Autodesk Inventor part; units mm, degrees
ref_plane "NUT_XY" through (0, 0, 0) normal (0, 0, 1) x (1, 0, 0)
ref_plane "NUT_YZ" through (0, 0, 0) normal (1, 0, 0) x (0, 1, 0)
ref_plane "NUT_ZX" through (0, 0, 0) normal (0, 1, 0) x (0, 0, 1)
sketch "Sketch_8" plane through (0, 0, 0) normal (1, 0, 0) x (0, 1, 0)
  line L0 (0, -3.048) -> (0, 0)
  line L1 (0, 0) -> (4.7625, 0)
  line L2 (4.7625, 0) -> (5.715, -0.2552)
  line L3 (5.715, -0.2552) -> (5.715, -2.7928)
  line L4 (5.715, -2.7928) -> (4.7625, -3.048)
  line L5 (4.7625, -3.048) -> (0, -3.048)
  line L6 (0, -3.048) -> (0, 0)
sketch "Sketch_10" plane through (0, 0, 0) normal (0, 0, 1) x (1, 0, 0)
  line L0 (-9.525, -9.525) -> (9.525, -9.525)
  line L1 (9.525, -9.525) -> (9.525, 9.525)
  line L2 (9.525, 9.525) -> (-9.525, 9.525)
  line L3 (-9.525, 9.525) -> (-9.525, -9.525)
  line L4 (-4.7625, -2.7496) -> (0, -5.4993)
  line L5 (0, -5.4993) -> (4.7625, -2.7496)
  line L6 (4.7625, -2.7496) -> (4.7625, 2.7496)
  line L7 (4.7625, 2.7496) -> (0, 5.4993)
  line L8 (0, 5.4993) -> (-4.7625, 2.7496)
  line L9 (-4.7625, 2.7496) -> (-4.7625, -2.7496)
revolve "Revolution1" add sketch "Sketch_8" angle 360 about axis through (0, 0, -3.048) along (0, 0, -1)
extrude "Extrusion1" cut sketch "Sketch_10" against normal blind 3.048
sketch "Sketch_11" plane through (0, 0, 0) normal (1, 0, 0) x (0, 1, 0)
  line L0 (0, -3.048) -> (0, 0)
  line L1 (0, 0) -> (2.413, 0)
  line L2 (2.413, 0) -> (1.9837, -0.4293)
  line L3 (1.9837, -0.4293) -> (1.9837, -2.6187)
  line L4 (1.9837, -2.6187) -> (2.413, -3.048)
  line L5 (2.413, -3.048) -> (0, -3.048)
  line L6 (0, -3.048) -> (0, 0)
revolve "Revolution2" cut sketch "Sketch_11" angle 360 about axis through (0, 0, -3.048) along (0, 0, -1)
thread "Thread1"
ref_plane "NUT_XY" through (0, 0, 0) normal (0, 0, 1) x (1, 0, 0)
ref_plane "NUT_YZ" through (0, 0, 0) normal (1, 0, 0) x (0, 1, 0)
ref_plane "NUT_ZX" through (0, 0, 0) normal (0, 1, 0) x (0, 0, 1)
ref_plane "a1_XY" through (-4.7625, 4.7625, 0) normal (0, 0, 1) x (1, 0, 0)
ref_plane "a1_YZ" through (-4.7625, 4.7625, 0) normal (1, 0, 0) x (0, 1, 0)
ref_plane "a1_ZX" through (-4.7625, 4.7625, 0) normal (0, 1, 0) x (0, 0, 1)
ref_plane "a2_XY" through (4.7625, 4.7625, 0) normal (0, 0, 1) x (1, 0, 0)
ref_plane "a2_YZ" through (4.7625, 4.7625, 0) normal (1, 0, 0) x (0, 1, 0)
ref_plane "a2_ZX" through (4.7625, 4.7625, 0) normal (0, 1, 0) x (0, 0, 1)
ref_plane "b1_XY" through (0, 4.7625, 0) normal (1, 0, 0) x (0, 0, -1)
ref_plane "b1_YZ" through (0, 4.7625, 0) normal (0, 0, -1) x (0, 1, 0)
ref_plane "b1_ZX" through (0, 4.7625, 0) normal (0, 1, 0) x (1, 0, 0)
ref_plane "b2_XY" through (0, 4.7625, -3.048) normal (1, 0, 0) x (0, 0, -1)
ref_plane "b2_YZ" through (0, 4.7625, -3.048) normal (0, 0, -1) x (0, 1, 0)
ref_plane "b2_ZX" through (0, 4.7625, -3.048) normal (0, 1, 0) x (1, 0, 0)
ref_plane "e_XY" through (0, 0, -3.048) normal (1, 0, 0) x (0, 0, -1)
ref_plane "e_YZ" through (0, 0, -3.048) normal (0, 0, -1) x (0, 1, 0)
ref_plane "e_ZX" through (0, 0, -3.048) normal (0, 1, 0) x (1, 0, 0)
ref_plane "ol1_XY" through (0, 0, -4.7625) normal (0, 1, 0) x (1, 0, 0)
ref_plane "ol1_YZ" through (0, 0, -4.7625) normal (1, 0, 0) x (0, 0, -1)
ref_plane "ol1_ZX" through (0, 0, -4.7625) normal (0, 0, -1) x (0, 1, 0)
ref_plane "ol2_XY" through (3.048, 0, -4.7625) normal (0, 1, 0) x (1, 0, 0)
ref_plane "ol2_YZ" through (3.048, 0, -4.7625) normal (1, 0, 0) x (0, 0, -1)
ref_plane "ol2_ZX" through (3.048, 0, -4.7625) normal (0, 0, -1) x (0, 1, 0)
ref_plane "th1_XY" through (0, 2.413, -3.048) normal (1, 0, 0) x (0, 0, -1)
ref_plane "th1_YZ" through (0, 2.413, -3.048) normal (0, 0, -1) x (0, 1, 0)
ref_plane "th1_ZX" through (0, 2.413, -3.048) normal (0, 1, 0) x (1, 0, 0)
ref_plane "th2_XY" through (0, -2.413, -3.048) normal (1, 0, 0) x (0, 0, -1)
ref_plane "th2_YZ" through (0, -2.413, -3.048) normal (0, 0, -1) x (0, 1, 0)
ref_plane "th2_ZX" through (0, -2.413, -3.048) normal (0, 1, 0) x (1, 0, 0)
properties part number "D-5288"
CAD build for the part. Positions are in the model's coordinates, mm. Coordinates: 2 decimals unless noted, no trailing zeros. Order: outer loops, then holes, each group sorted by start corner. A loop starts at its lowest first (then second) coordinate and runs counter-clockwise, first axis right, second up. Notation, with made-up numbers: M -31,44 L 7,44 A15 ccw 7,73 Z; hole C -4,-33.5 d3. An arc over 180 degrees is marked long. Answer as CSV lines item,"result".
1) Cut at A-A (z = -1.35). List the corners of the cut face in (x, y), then the cut area to 3 significant figures.
Verdict:
outline,"M -4.76,-2.75 L 0,-5.5 L 4.76,-2.75 L 4.76,2.75 L 0,5.5 L -4.76,2.75 Z; hole C 0,0 d3.97"
area,"66.2 mm2"
2) Mould opens along X. For faces 1 (the conical face through (-0.01, -4.94, -3)), 2 (the cylindrical face through (1.3, -1.5, -1.5)), 3 (the conical face through (-4.27, 2.48, -3)) say: released by +X, released by -X, zero draft, split by the parting line, or undercut.
Verdict:
face 1,"split by the parting line"
face 2,"undercut"
face 3,"released by -X"
3) Flat gauge pins, fed straight in: P1, Ø3.5, axis at x = 0, y = 0, coming from the +Z side; P2, Ø1, axis at x = -2, z = -2.5, coming from the +Y side. Where does each tip first touch, or does it go through?
Verdict:
P1,"through"
P2,"y = 4.63"
4) Drill centre lines: L1, parallel to X at y = 0, z = -1.4; L2, parallel to X at y = -1.75, z = -1.8; L3, parallel to Y at x = -0.5, z = -0.55. Where is each one in solid material? Low to high. Write a range as from..to.
Verdict:
L1,"-4.76..-1.98, 1.98..4.76"
L2,"-4.76..-0.93, 0.93..4.76"
L3,"-5.21..-1.92, 1.92..5.21"
